Source: CAD feature listing. Evaluate the final solid. Frame: model axes, mm. Coordinates: 2 decimals unless noted, no trailing zeros. Order: outer loops, then holes, each group sorted by start corner. A loop starts at its lowest first (then second) coordinate and runs counter-clockwise, first axis right, second up.
Item 1: Section C-C on z = 4.25. Return the cut outline in (x, y).
Item 2: Contact query for flat-ended pins moving along their axis: P1, Ø4.5, axis at x = 0, y = 15.47, coming from the -Z side; P2, Ø6.5, axis at y = 142, z = 8.5, coming from the -X side; P3, Ø2.5, axis at x = -9.5, y = 89, coming from the -Z side; P4, Ø3, axis at y = 220.5, z = 13, coming from the -X side. Output: stop coordinate, or through.
Item 3: Ray query, line 1 (Y direction, x = 0, z = 5.25); line 2 (Y direction, x = 0.5, z = 12.75); line 3 (X direction, y = 261.5, z = 2). Return the intervals inside material, ascending.
Item 4: Section A-A on x = 0.5. Return the cut outline in (y, z), then the cut area to 3 significant figures.
Item 5: Section B-B on y = 222. Return the cut outline in (x, z).
from build123d import *

# Parameters (mm, degrees)
F1_DEPTH = 355.6
F2_R     = 6.75023
F2_R_2   = 4.051718
F3_DEPTH = 5.08
F4_R     = 3.621045
F5_DEPTH = 25.4


with BuildPart() as f1:
    # F0 (on Front) → F1 (new body)
    with BuildSketch(Plane.XZ):
        with BuildLine():
            Line((10.668, 17.78), (0, 17.78))
            Line((0, 17.78), (-10.668, 17.78))
            ThreePointArc((-10.668, 17.78), (-12.104841, 17.184841), (-12.7, 15.748))
            Line((-12.7, 15.748), (-12.7, 14.732))
            ThreePointArc((-12.7, 14.732), (-12.104841, 13.295159), (-10.668, 12.7))
            Line((-10.668, 12.7), (-7.62, 12.7))
            Line((-7.62, 12.7), (-7.62, 0))
            Line((-7.62, 0), (0, 0))
            Line((0, 0), (7.62, 0))
            Line((7.62, 0), (7.62, 12.7))
            Line((7.62, 12.7), (10.668, 12.7))
            ThreePointArc((10.668, 12.7), (12.104841, 13.295159), (12.7, 14.732))
            Line((12.7, 14.732), (12.7, 15.748))
            ThreePointArc((12.7, 15.748), (12.104841, 17.184841), (10.668, 17.78))
        make_face()
    extrude(amount=-F1_DEPTH)

    # F2 (on face) → F3 (cut)
    with BuildSketch(Plane.XY.offset(17.78)):
        with Locations((0, 15.474608)):
            Circle(F2_R)
        with Locations((0, 15.474608)):
            Circle(F2_R_2, mode=Mode.SUBTRACT)
        with Locations((0, 15.474608)):
            Circle(F2_R_2)
    extrude(amount=-F3_DEPTH, mode=Mode.SUBTRACT)

    # F4 (on face) → F5 (cut)
    with BuildSketch(Plane.XY.offset(17.78)):
        with Locations((0, 15.474608)):
            Circle(F4_R)
    extrude(amount=-F5_DEPTH, mode=Mode.SUBTRACT)


solid = f1.part
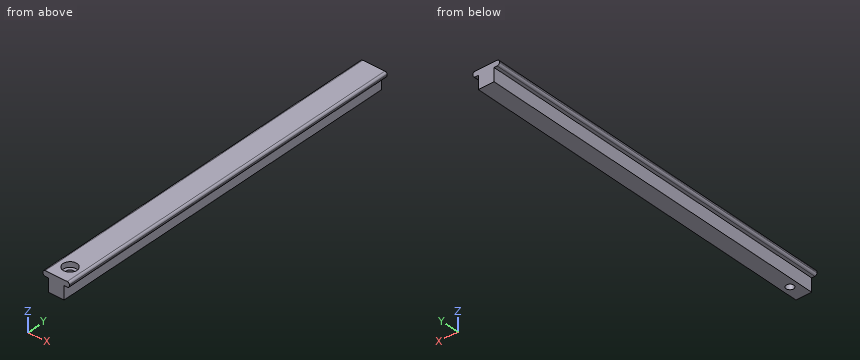
Answer list:
1. outline: (-7.62, 0) - (7.62, 0) - (7.62, 355.6) - (-7.62, 355.6) - close; hole circle Ø7.24 at (0, 15.47)
2. P1: passes through
2. P2: stops at x = -7.62
2. P3: stops at z = 12.7
2. P4: stops at x = -12.69
3. line 1: y = 0 to 11.85, 19.1 to 355.6
3. line 2: y = 0 to 8.74, 22.21 to 355.6
3. line 3: x = -7.62 to 7.62
4. outline: (0, 0) - (11.89, 0) - (11.89, 12.7) - (8.74, 12.7) - (8.74, 17.78) - (0, 17.78) - close; (19.06, 0) - (355.6, 0) - (355.6, 17.78) - (22.21, 17.78) - (22.21, 12.7) - (19.06, 12.7) - close
4. area: 6,160 mm2
5. outline: (-12.7, 14.73) arc R2.03 ccw to (-10.67, 12.7) - (-7.62, 12.7) - (-7.62, 0) - (7.62, 0) - (7.62, 12.7) - (10.67, 12.7) arc R2.03 ccw to (12.7, 14.73) - (12.7, 15.75) arc R2.03 ccw to (10.67, 17.78) - (-10.67, 17.78) arc R2.03 ccw to (-12.7, 15.75) - close
